Can you work these out from the model? Positions are in its coordinate system, mm. A direction names the side the tool comes from. Round coordinates to 2 decimals unless told otherwise and drop trailing zeros. Loops run counter-clockwise (first coordinate to the right, second up) from the corner with the lowest first, then second, coordinate; pieces in that order, holes last. Notation, with made-up numbers: (-13, 5) - (44, 5) arc R36 ccw to (44, 44) - close; hole circle Ø1 at (32.25, 11.5). An arc over 180 degrees is marked (long way). Answer as CSV lines item,"result".
```python
from build123d import *

# Parameters (mm, degrees)
F1_DEPTH = 2
F2_DEPTH = 2


with BuildPart() as f1:
    # F0 (on Front) → F1 (new body, symmetric)
    with BuildSketch(Plane.XZ):
        with BuildLine():
            Line((16.5, 3), (0, 3))
            Line((0, 3), (-16.5, 3))
            ThreePointArc((-16.5, 3), (-19.446852, 3.054649), (-21.916025, 4.664031))
            ThreePointArc((-21.916025, 4.664031), (-26.681772, 8.233743), (-32.5, 9.5))
            Line((-32.5, 9.5), (-57.5, 9.5))
            Line((-57.5, 9.5), (-57.5, -9.5))
            Line((-57.5, -9.5), (-32.5, -9.5))
            ThreePointArc((-32.5, -9.5), (-26.681772, -8.233743), (-21.916025, -4.664031))
            ThreePointArc((-21.916025, -4.664031), (-19.446852, -3.054649), (-16.5, -3))
            Line((-16.5, -3), (0, -3))
            Line((0, -3), (16.5, -3))
            ThreePointArc((16.5, -3), (19.446852, -3.054649), (21.916025, -4.664031))
            ThreePointArc((21.916025, -4.664031), (26.681772, -8.233743), (32.5, -9.5))
            Line((32.5, -9.5), (57.5, -9.5))
            Line((57.5, -9.5), (57.5, 9.5))
            Line((57.5, 9.5), (32.5, 9.5))
            ThreePointArc((32.5, 9.5), (26.681772, 8.233743), (21.916025, 4.664031))
            ThreePointArc((21.916025, 4.664031), (19.446852, 3.054649), (16.5, 3))
        make_face()
    extrude(amount=F1_DEPTH, both=True)

    # F0 (on Front) → F2 (join, symmetric)
    with BuildSketch(Plane.XZ):
        with BuildLine():
            Line((16.5, 3), (0, 3))
            Line((0, 3), (-16.5, 3))
            ThreePointArc((-16.5, 3), (-19.446852, 3.054649), (-21.916025, 4.664031))
            ThreePointArc((-21.916025, 4.664031), (-26.681772, 8.233743), (-32.5, 9.5))
            Line((-32.5, 9.5), (-57.5, 9.5))
            Line((-57.5, 9.5), (-57.5, -9.5))
            Line((-57.5, -9.5), (-32.5, -9.5))
            ThreePointArc((-32.5, -9.5), (-26.681772, -8.233743), (-21.916025, -4.664031))
            ThreePointArc((-21.916025, -4.664031), (-19.446852, -3.054649), (-16.5, -3))
            Line((-16.5, -3), (0, -3))
            Line((0, -3), (16.5, -3))
            ThreePointArc((16.5, -3), (19.446852, -3.054649), (21.916025, -4.664031))
            ThreePointArc((21.916025, -4.664031), (26.681772, -8.233743), (32.5, -9.5))
            Line((32.5, -9.5), (57.5, -9.5))
            Line((57.5, -9.5), (57.5, 9.5))
            Line((57.5, 9.5), (32.5, 9.5))
            ThreePointArc((32.5, 9.5), (26.681772, 8.233743), (21.916025, 4.664031))
            ThreePointArc((21.916025, 4.664031), (19.446852, 3.054649), (16.5, 3))
        make_face()
    extrude(amount=F2_DEPTH, both=True)


solid = f1.part
```
Q1. I'm going to push a flat-ended pin straight in: pin 1 Ø5 at (x, z) = (10.5, 6) entering from +Y. Where does the tip first touch, or does it pass through?
Checks:
pin 1,"through"
Q2. Imagine slicing it at A-A (z = 6). Write out the boundary of the cut face in (x, y), then the cut area to 3 significant figures.
Checks:
outline,"(-57.5, -2) - (-23.24, -2) - (-23.24, 2) - (-57.5, 2) - close; (23.24, -2) - (57.5, -2) - (57.5, 2) - (23.24, 2) - close"
area,"274 mm²"
Q3. We'd pull the mould along X, two halves only. Please class faces 4 (the flat face through (-1, -2, 0)), 5 (the cylindrical face through (19.49, -0.03, 3.07)), 6 (the flat face through (-57.5, 0, 0)), 7 (the cylindrical face through (-26.61, -0.03, 8.2)): pulls with the +X half, pulls with the -X half, needs draft (parallel to the pull), parting line crosses it, or undercut.
Checks:
face 4,"needs draft"
face 5,"undercut"
face 6,"pulls with the -X half"
face 7,"undercut"
Q4. Imagine slicing it at B-B (y = -0.65). Write out the boundary of the cut face in (x, z), then the cut area to 3 significant figures.
Checks:
outline,"(-57.5, -9.5) - (-32.5, -9.5) arc R14 ccw to (-21.92, -4.66) arc R5.34 cw to (-16.5, -3) - (16.5, -3) arc R5.34 cw to (21.92, -4.66) arc R14 ccw to (32.5, -9.5) - (57.5, -9.5) - (57.5, 9.5) - (32.5, 9.5) arc R14 ccw to (21.92, 4.66) arc R5.34 cw to (16.5, 3) - (-16.5, 3) arc R5.34 cw to (-21.92, 4.66) arc R14 ccw to (-32.5, 9.5) - (-57.5, 9.5) - close"
area,"1,560 mm²"
Q5. If I drill on line 1 along X through (y, z) = (-0.9, -7.25); line 2 along Z through (x, y) = (13.5, 1.35); line 3 along X through (y, z) = (1.3, -3.25), over which ranges is the centre line in solid material (lowest first)? Write a range as [from, to].
Checks:
line 1,"[-57.5, -24.89], [24.89, 57.5]"
line 2,"[-3, 3]"
line 3,"[-57.5, -19.98], [19.98, 57.5]"
Q6. On a 3-axis mill with a long thin cutter (end or side, diameter ignored), from which of +Z, -Z, +X, -X, +Y, -Y can I reach the whole of each face in a straight line? I mean faces 1 (the cylindrical face through (26.76, -0.03, 8.27)), 2 (the cylindrical face through (26.61, -0.03, -8.2)), 3 (the flat face through (45, 0, -9.5)). Say none if no direction works.
Checks:
face 1,"+Z, +Y, -Y"
face 2,"-Z, +Y, -Y"
face 3,"-Z, +X, -X, +Y, -Y"
Q7. Imagine slicing it at C-C (x = 5.5). Write out the boundary of the cut face in (y, z), then the cut area to 3 significant figures.
Checks:
outline,"(-2, -3) - (2, -3) - (2, 3) - (-2, 3) - close"
area,"24.0 mm²"
Q8. Imagine slicing it at D-D (z = -7). Write out the boundary of the cut face in (x, y).
Checks:
outline,"(-57.5, -2) - (-24.52, -2) - (-24.52, 2) - (-57.5, 2) - close; (24.52, -2) - (57.5, -2) - (57.5, 2) - (24.52, 2) - close"
